Could you check a few things on this model? Use its own coordinates, in mm. Face numbers are marked on the shaded views. A direction names the side the tool comes from. Round coordinates to 2 decimals unless told otherwise and drop trailing zeros. Order: outer loops, then holes, each group sorted by start corner. A loop starts at its lowest first (then second) coordinate and runs counter-clockwise, first axis right, second up. Notation, with made-up numbers: (-29, 17) - (0, 17) arc R19 cw to (0, 39) - close; hole circle Ø9 at (-36, -39.75). An arc over 180 degrees is marked (long way). Use one line per item in the form item = value.
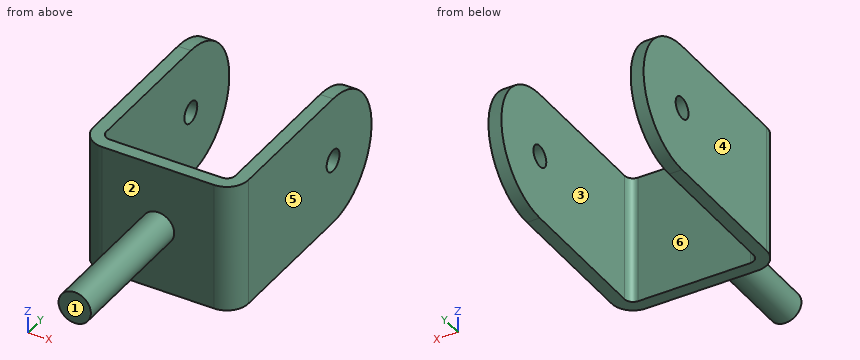
from build123d import *
from build123d.topology import SkipClean

# Parameters (mm, degrees)
BOSS_EXTRUDE1_DEPTH = 300
SKETCH2_R           = 37.5
BOSS_EXTRUDE2_DEPTH = 325
BOSS_EXTRUDE3_DEPTH = 30
SKETCH3_4_R         = 25
CUT_EXTRUDE1_DEPTH  = 360
BOSS_EXTRUDE4_START = -30
BOSS_EXTRUDE4_DEPTH = 30
SKETCH3_9_R         = 25
CUT_EXTRUDE2_DEPTH  = 360


with BuildPart() as part:
    # Sketch1 → Boss-Extrude1 (new body)
    with BuildSketch(Plane.XY):
        with BuildLine():
            Line((-130, 0), (130, 0))
            ThreePointArc((130, 0), (165.355339059, 14.644660941), (180, 50))
            Line((180, 50), (180, 380))
            Line((180, 380), (150, 380))
            Line((150, 380), (150, 50))
            ThreePointArc((150, 50), (144.142135624, 35.857864376), (130, 30))
            Line((130, 30), (-130, 30))
            ThreePointArc((-130, 30), (-144.142135624, 35.857864376), (-150, 50))
            Line((-150, 50), (-150, 380))
            Line((-150, 380), (-180, 380))
            Line((-180, 380), (-180, 50))
            ThreePointArc((-180, 50), (-165.355339059, 14.644660941), (-130, 0))
        make_face()
    extrude(amount=BOSS_EXTRUDE1_DEPTH)

    # Sketch2 → Boss-Extrude2 (add)
    with BuildSketch(Plane.XZ):
        with Locations(Location((0, 150, 0), (0, 0, 90))):
            Circle(SKETCH2_R)
    extrude(amount=BOSS_EXTRUDE2_DEPTH)

    # Sketch3 → Boss-Extrude3 (add)
    with BuildSketch(Plane(origin=(180, 0, 0), x_dir=(0, 0, -1), z_dir=(1, 0, 0))):
        with BuildLine():
            ThreePointArc((0, 380), (-150, 530), (-300, 380))
            Line((-300, 380), (-175, 380))
            ThreePointArc((-175, 380), (-150, 405), (-125, 380))
            Line((-125, 380), (0, 380))
        make_face()
    extrude(amount=-BOSS_EXTRUDE3_DEPTH)

    # Sketch3<4> → Cut-Extrude1 (cut)
    with SkipClean():  # the faces are left unmerged after this step: merging them gives an invalid solid
        with BuildSketch(Plane(origin=(180, 0, 0), x_dir=(0, 0, -1), z_dir=(1, 0, 0))):
            with Locations(Location((-150, 380, 0), (0, 0, 90))):
                Circle(SKETCH3_4_R)
        extrude(amount=-CUT_EXTRUDE1_DEPTH, mode=Mode.SUBTRACT)

    # Sketch6 → Boss-Extrude4 (add)
    with BuildSketch(Plane.ZY.offset(180).offset(BOSS_EXTRUDE4_START)):
        with BuildLine():
            Line((0, 380), (0, 50))
            Line((0, 50), (300, 50))
            Line((300, 50), (300, 380))
            ThreePointArc((300, 380), (150, 530), (0, 380))
        make_face()
    extrude(amount=BOSS_EXTRUDE4_DEPTH)

    # Sketch3<9> → Cut-Extrude2 (cut)
    with BuildSketch(Plane(origin=(180, 0, 0), x_dir=(0, 0, -1), z_dir=(1, 0, 0))):
        with Locations(Location((-150, 380, 0), (0, 0, 90))):
            Circle(SKETCH3_9_R)
    extrude(amount=-CUT_EXTRUDE2_DEPTH, mode=Mode.SUBTRACT)


solid = part.part
Item 1: For the marked faces 1, 2 and 3, which set-ups out of +Z, -Z, +X, -X, +Y, -Y let a thin tool reach every point of the face, with its end or its side?
Found:
face_1 = +Z, -Z, +X, -X, -Y
face_2 = -Y
face_3 = +Z, -Z, +Y
Item 2: If we mould it in two halves opening along X, with no side actions, what happens to the marked faces 4, 5 and 6? For each: released by +X, released by -X, zero draft, split by the parting line, or undercut.
Found:
face_4 = released by -X
face_5 = released by +X
face_6 = undercut
Item 3: Imagine slicing it at A-A on z = 150. Please give me the cut outline in (x, y), plus the area to 3 significant figures.
Found:
outline = (-180, 50) arc R50 ccw to (-130, 0) - (-37.5, 0) - (-37.5, -325) - (37.5, -325) - (37.5, 0) - (130, 0) arc R50 ccw to (180, 50) - (180, 355) - (150, 355) - (150, 50) arc R20 cw to (130, 30) - (-130, 30) arc R20 cw to (-150, 50) - (-150, 355) - (-180, 355) - close; (-180, 405) - (-150, 405) - (-150, 530) - (-180, 530) - close; (150, 405) - (180, 405) - (180, 530) - (150, 530) - close
area = 61,300 mm2
Item 4: Imagine slicing it at B-B on y = 244. Please give me the cut outline in (x, z), plus the area to 3 significant figures.
Found:
outline = (-180, 0) - (-150, 0) - (-150, 300) - (-180, 300) - close; (150, 0) - (180, 0) - (180, 300) - (150, 300) - close
area = 18,000 mm2
Item 5: Will these pins go through, and if not, where does the flat tip stop? P1, Ø12, axis at x = 55, z = 235.5, coming from the -Y side; P2, Ø12, axis at x = -142.5, z = 264, coming from the -Y side; P3, Ø10, axis at y = -145.5, z = 114.5, coming from the -X side.
Found:
P1 = 0
P2 = 0.42
P3 = -21.82
Item 6: I need wall thicknesses on L1, parallel to X at y = 469.5, z = 80; L2, parallel to Z at x = -158.75, y = 380; L3, parallel to Y at x = 33.5, z = 155.5. Which ranges of each line are inside material? Lowest first, please.
Found:
L1 = -180 to -150, 150 to 180
L2 = 0 to 125, 175 to 300
L3 = -325 to 30
Item 7: Imagine slicing it at C-C on x = 0. Please give me the cut outline in (y, z).
Found:
outline = (-325, 112.5) - (0, 112.5) - (0, 0) - (30, 0) - (30, 300) - (0, 300) - (0, 187.5) - (-325, 187.5) - close
Item 8: Imagine slicing it at D-D on y = 440. Please give me the cut outline in (x, z).
Found:
outline = (-180, 12.52) - (-150, 12.52) - (-150, 287.48) - (-180, 287.48) - close; (150, 12.52) - (180, 12.52) - (180, 287.48) - (150, 287.48) - close
